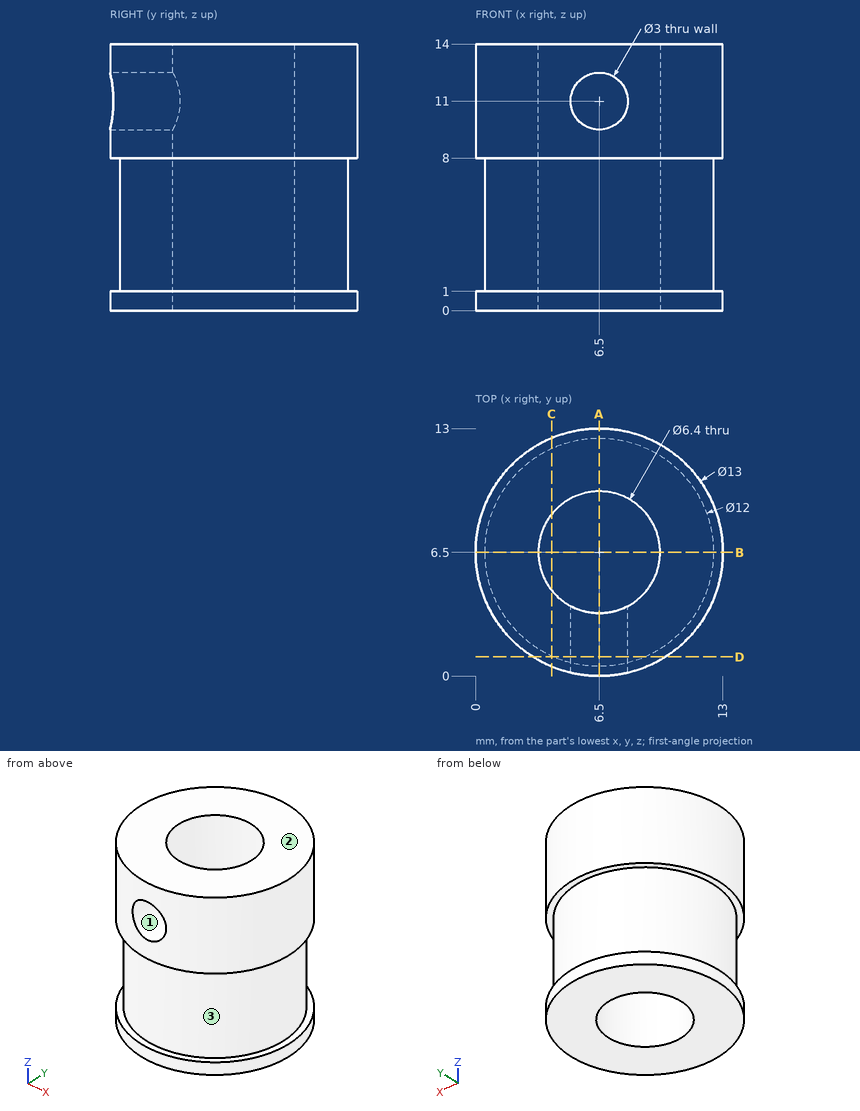
Answer from the drawing. Dimensions are ordinates in mm from the lowest x, y and z of the part. Give positions to 0.01 mm unless a question says otherwise; leave off trailing zeros. Order: outer loops, then holes, each group sorted by start corner. A loop starts at its lowest first (then second) coordinate and runs counter-clockwise, first axis right, second up. Notation, with made-up numbers: (-22.5, 29) - (-8.5, 29) arc R17 cw to (-8.5, 38) - close; hole circle Ø4 at (50.25, 81.25). An arc over 180 degrees is marked (long way). One line per item, written item: value. Start each with the question number.
1) A cutting plane is placed at A-A on x = 6.5. Give the vertices of the cut face in (y, z).
2) A cutting plane is placed at D-D on y = 1. Give the vertices of the cut face in (x, z), then the cut area to 3 significant figures.
3) The mould has two halves that part along X. Classify the marked faces 1, 2 and 3: released by +X, released by -X, zero draft, split by the parting line, or undercut.
4) A cutting plane is placed at C-C on x = 4. Give the vertices of the cut face in (y, z), then the cut area to 3 significant figures.
5) Given pin 1 Ø6 at (x, y) = (6.5, 6.5) entering from +Z; pin 2 Ø1.5 at (y, z) = (10, 3) entering from +X; pin 3 Ø3 at (x, z) = (9, 1.5) entering from +Y, each flat-ended and moving along its own axis, determine where each tip first touches the part or whether it passes through.
6) Find the intervals of material crossed by L1, parallel to Z at x = 12.25, y = 8.5; L2, parallel to Y at x = 6.5, z = 7; L3, parallel to Y at x = 8.5, z = 4, in increasing order.
7) A cutting plane is placed at B-B on y = 6.5. Give the vertices of the cut face in (x, z), then the cut area to 3 significant figures.
Answer sheet:
1. outline: (0, 0) - (3.3, 0) - (3.3, 9.5) - (0, 9.5) - (0, 8) - (0.5, 8) - (0.5, 1) - (0, 1) - close; (0, 12.5) - (3.3, 12.5) - (3.3, 14) - (0, 14) - close; (9.7, 0) - (13, 0) - (13, 1) - (12.5, 1) - (12.5, 8) - (13, 8) - (13, 14) - (9.7, 14) - close
2. outline: (3.04, 0) - (9.96, 0) - (9.96, 1) - (8.9, 1) - (8.9, 8) - (9.96, 8) - (9.96, 14) - (3.04, 14) - (3.04, 8) - (4.1, 8) - (4.1, 1) - (3.04, 1) - close; hole circle Ø3 at (6.5, 11)
2. area: 75.0 mm2
3. face 1: undercut
3. face 2: zero draft
3. face 3: split by the parting line
4. outline: (0.5, 0) - (4.5, 0) - (4.5, 14) - (0.5, 14) - (0.5, 8) - (1.05, 8) - (1.05, 1) - (0.5, 1) - close; (8.5, 0) - (12.5, 0) - (12.5, 1) - (11.95, 1) - (11.95, 8) - (12.5, 8) - (12.5, 14) - (8.5, 14) - close
4. area: 104 mm2
5. pin 1: passes through
5. pin 2: stops at x = 11.83
5. pin 3: stops at y = 12.91
6. L1: z = 0 to 1, 8 to 14
6. L2: y = 0.5 to 3.3, 9.7 to 12.5
6. L3: y = 0.84 to 4, 9 to 12.16
7. outline: (0, 0) - (3.3, 0) - (3.3, 14) - (0, 14) - (0, 8) - (0.5, 8) - (0.5, 1) - (0, 1) - close; (9.7, 0) - (13, 0) - (13, 1) - (12.5, 1) - (12.5, 8) - (13, 8) - (13, 14) - (9.7, 14) - close
7. area: 85.4 mm2
